Read the model definition and answer for the solid it produces. Units are mm, in the model's axes. A direction names the side the tool comes from. Give positions to 0.01 mm unless a question says otherwise; leave off trailing zeros. Loops run counter-clockwise (first coordinate to the right, second up) from the corner with the lowest first, then second, coordinate; pieces in that order, holes last. Notation, with made-up numbers: (51, 25) - (73, 25) arc R19 ccw to (73, 57) - close; hole circle Ø4 at (14, 58). An arc over 180 degrees is marked (long way). Write each question's results on one line, items separated by ' | '. Start each with the question number.
Q1. The part is cut by section A-A, the plane z = 0. Write down the section's boundary in (x, y).
Q2. The part is cut by section D-D, the plane z = -107. Write down the section's boundary in (x, y).
Q3. For faces 4 (the flat face through (0, 33, 5.737)), 5 (the flat face through (0, 2, 0)), 6 (the cylindrical face through (-4.396, 1.521, -1.593)), 7 (the flat face through (-2, 52, -113.948)), determine the directions among +Z, -Z, +X, -X, +Y, -Y from which every point of the face is accessible in a straight line to the end or side of a thin tool.
Q4. Given pin 1 (4 mm diameter, centred on x = 4.5, z = -71.5, fed in from -Y); pin 2 (1 mm diameter, centred on x = 2.5, z = -115, fed in from -Y); pin 3 (2 mm diameter, centred on x = -1, y = 1, fed in from -Z), each flat-ended and moving along its own axis, determine where each tip first touches the part or whether it passes through.
Q5. The part is cut by section B-B, the plane x = 0. Write down the section's boundary in (y, z).
Q6. The part is cut by section C-C, the plane y = 25.5. Write down the section's boundary in (x, z).
Q7. Find the intervals of material crossed by line 1 (X direction, y = 1.75, z = 0); line 2 (Z direction, x = -8, y = 50.5); line 3 (Y direction, x = 5.5, z = -107.5), in increasing order. Write a range as from..to.
Q8. Determine the mould class of faces 1 (the flat face through (0, 64.15, -55)), 2 (the cylindrical face through (0.176, 51.917, -114.962)), 3 (the flat face through (-8.75, 65, -49)) for opening direction X: +X half, -X half, draft (parallel to the pull), parting line (faces both ways), or undercut.
```python
from build123d import *

# Parameters (mm, degrees)
SKETCH1_W                                         = 17.5
SKETCH1_H                                         = 10
BASE_FLANGE1_DEPTH                                = 2
EDGE_FLANGE1_DEPTH                                = 17.5
EDGE_FLANGE2_STRIP_W                              = 9.4732
EDGE_FLANGE2_STRIP_H                              = 2
EDGE_FLANGE2_STRIP_CUT_DEPTH                      = 17.5
EDGE_FLANGE2_DEPTH                                = 17.5
EDGE_FLANGE3_STRIP_W                              = 9.4732
EDGE_FLANGE3_STRIP_H                              = 2
EDGE_FLANGE3_STRIP_CUT_DEPTH                      = 17.5
EDGE_FLANGE3_DEPTH                                = 17.5
SKETCH18_R                                        = 4
CUT_EXTRUDE2_DEPTH                                = 2
CSK_FOR_4_FLAT_HEAD_MACHINE_SCREW_100_D           = 3.2639
CSK_FOR_4_FLAT_HEAD_MACHINE_SCREW_100_DEPTH       = 2
CSK_FOR_4_FLAT_HEAD_MACHINE_SCREW_100_CSINK_D     = 5.715
CSK_FOR_4_FLAT_HEAD_MACHINE_SCREW_100_CSINK_ANGLE = 100
CSK_FOR_4_FLAT_HEAD_MACHINE_SCREW_100_TIP         = 0.980574487


# Sheet-metal steps are written as plain solids
with BuildPart() as part:
    # Sketch1 → Base-Flange1 (new body)
    with BuildSketch(Plane(origin=(0, 0, 0), x_dir=(1, 0, 0), z_dir=(0, 1, 0))):
        Rectangle(SKETCH1_W, SKETCH1_H)
    extrude(amount=BASE_FLANGE1_DEPTH)

    # Edge-Flange1 section (across the edge) → Edge-Flange1 (add)
    with BuildSketch(Plane(origin=(-8.75, 2, 5.7366), x_dir=(0, 0, -1), z_dir=(1, 0, 0))):
        with BuildLine():
            Line((-2, 0.7366), (-2, 64.15))
            Line((-2, 64.15), (0, 64.15))
            Line((0, 64.15), (0, 0.7366))
            ThreePointArc((0, 0.7366), (0.215745145, 0.215745145), (0.7366, 0))
            Line((0.7366, 0), (0.7366, -2))
            ThreePointArc((0.7366, -2), (-1.198468417, -1.198468417), (-2, 0.7366))
        make_face()
    extrude(amount=EDGE_FLANGE1_DEPTH)

    # Edge-Flange2 strip (across the edge) → Edge-Flange2 strip cut (cut)
    with BuildSketch(Plane(origin=(-8.75, 66.15, 5.7366), x_dir=(0, -1, 0), z_dir=(1, 0, 0))):
        with Locations((-2, -1)):
            Rectangle(EDGE_FLANGE2_STRIP_W, EDGE_FLANGE2_STRIP_H)
    extrude(amount=EDGE_FLANGE2_STRIP_CUT_DEPTH, mode=Mode.SUBTRACT)

    # Edge-Flange2 section (across the edge) → Edge-Flange2 (add)
    with BuildSketch(Plane(origin=(-8.75, 66.15, 5.7366), x_dir=(0, -1, 0), z_dir=(1, 0, 0))):
        with BuildLine():
            Line((0, 0.7366), (0, 121.685))
            Line((0, 121.685), (2, 121.685))
            Line((2, 121.685), (2, 0.7366))
            ThreePointArc((2, 0.7366), (2.215745145, 0.215745145), (2.7366, 0))
            Line((2.7366, 0), (2.7366, -2))
            ThreePointArc((2.7366, -2), (0.801531583, -1.198468417), (0, 0.7366))
        make_face()
    extrude(amount=EDGE_FLANGE2_DEPTH)

    # Edge-Flange3 strip (across the edge) → Edge-Flange3 strip cut (cut)
    with BuildSketch(Plane(origin=(-8.75, 64.15, -115.9484), x_dir=(0, 0, 1), z_dir=(1, 0, 0))):
        with Locations((-2, -1)):
            Rectangle(EDGE_FLANGE3_STRIP_W, EDGE_FLANGE3_STRIP_H)
    extrude(amount=EDGE_FLANGE3_STRIP_CUT_DEPTH, mode=Mode.SUBTRACT)

    # Edge-Flange3 section (across the edge) → Edge-Flange3 (add)
    with BuildSketch(Plane(origin=(-8.75, 64.15, -115.9484), x_dir=(0, 0, 1), z_dir=(1, 0, 0))):
        with BuildLine():
            Line((0, 0.7366), (0, 16))
            Line((0, 16), (2, 16))
            Line((2, 16), (2, 0.7366))
            ThreePointArc((2, 0.7366), (2.215745145, 0.215745145), (2.7366, 0))
            Line((2.7366, 0), (2.7366, -2))
            ThreePointArc((2.7366, -2), (0.801531583, -1.198468417), (0, 0.7366))
        make_face()
    extrude(amount=EDGE_FLANGE3_DEPTH)

    # Sketch18 → Cut-Extrude2 (cut)
    with BuildSketch(Plane(origin=(0, 0, -115.9484), x_dir=(-1, 0, 0), z_dir=(0, 0, -1))):
        with Locations(Location((0, 55.9134, 0), (0, 0, 90))):
            Circle(SKETCH18_R)
    extrude(amount=-CUT_EXTRUDE2_DEPTH, mode=Mode.SUBTRACT)

    # CSK for #4 Flat Head Machine Screw (100)1
    with Locations(Plane.XZ):
        with Locations((4.75, 0), (-4.75, 0)):
            CounterSinkHole(CSK_FOR_4_FLAT_HEAD_MACHINE_SCREW_100_D / 2, CSK_FOR_4_FLAT_HEAD_MACHINE_SCREW_100_CSINK_D / 2, depth=CSK_FOR_4_FLAT_HEAD_MACHINE_SCREW_100_DEPTH, counter_sink_angle=CSK_FOR_4_FLAT_HEAD_MACHINE_SCREW_100_CSINK_ANGLE)
            with Locations((0, 0, -(CSK_FOR_4_FLAT_HEAD_MACHINE_SCREW_100_DEPTH + CSK_FOR_4_FLAT_HEAD_MACHINE_SCREW_100_TIP / 2))):  # 118° drill point
                Cone(0, CSK_FOR_4_FLAT_HEAD_MACHINE_SCREW_100_D / 2, CSK_FOR_4_FLAT_HEAD_MACHINE_SCREW_100_TIP, mode=Mode.SUBTRACT)


solid = part.part
```
Check sheet entries:
1) outline: (-8.75, 0) - (-7.61, 0) - (-6.38, 1.03) - (-6.38, 2) - (-8.75, 2) - close; (-8.75, 64.15) - (8.75, 64.15) - (8.75, 66.15) - (-8.75, 66.15) - close; (-3.12, 1.03) - (-1.89, 0) - (1.89, 0) - (3.12, 1.03) - (3.12, 2) - (-3.12, 2) - close; (6.38, 1.03) - (7.61, 0) - (8.75, 0) - (8.75, 2) - (6.38, 2) - close
2) outline: (-8.75, 64.15) - (8.75, 64.15) - (8.75, 66.15) - (-8.75, 66.15) - close
3) face 4: +X, -X | face 5: -Z, +X, -X | face 6: -Y | face 7: +X, -X, -Y
4) pin 1: stops at y = 64.15 | pin 2: stops at y = 48.15 | pin 3: stops at z = -5
5) outline: (0, -5) - (2, -5) - (2, 5) arc R0.74 cw to (2.74, 5.74) - (63.41, 5.74) arc R0.74 cw to (64.15, 5) - (64.15, -113.21) arc R0.74 cw to (63.41, -113.95) - (59.91, -113.95) - (59.91, -115.95) - (63.41, -115.95) arc R2.74 ccw to (66.15, -113.21) - (66.15, 5) arc R2.74 ccw to (63.41, 7.74) - (2.74, 7.74) arc R2.74 ccw to (0, 5) - close; (48.15, -115.95) - (51.91, -115.95) - (51.91, -113.95) - (48.15, -113.95) - close
6) outline: (-8.75, 5.74) - (8.75, 5.74) - (8.75, 7.74) - (-8.75, 7.74) - close
7) line 1: x = -8.75..-6.38, -3.12..3.12, 6.38..8.75 | line 2: z = -115.95..-113.95, 5.74..7.74 | line 3: y = 64.15..66.15
8) face 1: draft | face 2: undercut | face 3: -X half
